from build123d import *

# Parameters (mm, degrees)
F0_R     = 1.25
F1_DEPTH = 2
F2_W     = 20
F2_H     = 3.15
F3_DEPTH = 15
F4_R     = 9.99999
F5_R     = 2.55
F6_DEPTH = 25


# Not quite as in the source:
# - a fillet or chamfer is up to 0.001 mm smaller than in the source, because OpenCascade refuses the exact size


with BuildPart() as f1:
    # F0 (on Top) → F1 (new body)
    with BuildSketch(Plane.XY):
        with BuildLine():
            Line((-33, -15), (33, -15))
            ThreePointArc((33, -15), (34.4142135624, -14.4142135624), (35, -13))
            Line((35, -13), (35, 13))
            ThreePointArc((35, 13), (34.4142135624, 14.4142135624), (33, 15))
            Line((33, 15), (-33, 15))
            ThreePointArc((-33, 15), (-34.4142135624, 14.4142135624), (-35, 13))
            Line((-35, 13), (-35, -13))
            ThreePointArc((-35, -13), (-34.4142135624, -14.4142135624), (-33, -15))
        make_face()
        with Locations((-30.5, -12)):
            Circle(F0_R, mode=Mode.SUBTRACT)
        with Locations((30.5, -12)):
            Circle(F0_R, mode=Mode.SUBTRACT)
        with Locations((-30.5, 12)):
            Circle(F0_R, mode=Mode.SUBTRACT)
        with Locations((30.5, 12)):
            Circle(F0_R, mode=Mode.SUBTRACT)
    extrude(amount=F1_DEPTH)

    # F2 (on face) → F3 (join)
    with BuildSketch(Plane.XY.offset(2)):
        Rectangle(F2_W, F2_H)
        with Locations((0, 6.6)):
            Rectangle(F2_W, F2_H)
        with Locations((0, -6.6)):
            Rectangle(F2_W, F2_H)
    extrude(amount=F3_DEPTH)

    # F4 (radius 10 in the source; OpenCascade refuses exactly that, so slightly less here)
    f4_edges = [f1.edges().sort_by_distance(p)[0] for p in [
        (-10, -6.6, 17),
        (10, -6.6, 17),
        (10, 0, 17),
        (-10, 0, 17),
        (-10, 6.6, 17),
        (10, 6.6, 17),
    ]]
    fillet(f4_edges, radius=F4_R)

    # F5 (on face) → F6 (cut)
    with BuildSketch(Plane.XZ.offset(8.175)):
        with Locations((0, 12)):
            Circle(F5_R)
    extrude(amount=-F6_DEPTH, mode=Mode.SUBTRACT)


solid = f1.part
Work out the finished part from the listing and answer in its coordinate system (mm). A direction names the side the tool comes from. Round coordinates to 2 decimals unless told otherwise and drop trailing zeros. Loops run counter-clockwise (first coordinate to the right, second up) from the corner with the lowest first, then second, coordinate; pieces in that order, holes last. Notation, with made-up numbers: (35.25, 80.5) - (64.25, 80.5) arc R26 ccw to (64.25, 119.5) - close; hole circle Ø5 at (45.5, 2.5). An arc over 180 degrees is marked (long way). Use one line per item in the form item = value. Start each with the question number.
(1) Flat-ended cylindrical pins translate along their axes: P1, Ø4, axis at x = 7, y = 2, coming from the -Z side; P2, Ø4, axis at x = 0, z = 12, coming from the +Y side; P3, Ø8, axis at x = 14, y = 11, coming from the +Z side; P4, Ø3, axis at x = 11, z = 9.5, coming from the +Y side (3 decimals). Find the tip coordinate at first contact, or state that the pin passes through.
(2) Determine the mould class of faces 6 (the face through (0, -5.025, 8)), 7 (the face through (34.4, -14.43, 0.99)), 8 (the face through (7.15, 0.02, 13.99)) for opening direction Y: +Y half, -Y half, draft (parallel to the pull), parting line (faces both ways), or undercut.
(3) Find section B-B on z = 3. Determine the outline of the cut face in (x, y) (3 decimals), and give its area (3 significant figures).
(4) Consider line 1 (Y direction, x = -30.5, z = 1.1); line 2 (Y direction, x = -4, z = 9) (3 decimals); line 3 (Z direction, x = 0, y = 0). Determine where each line is inside the solid, lowest interval first.
(5) Which of the six approach directions +Z, -Z, +X, -X, +Y, -Y give full straight-line access (tool end or side, diameter ignored) to faces 1 (the face through (0, -15, 1)), 2 (the face through (-35, 0, 1)), 3 (the face through (-10, -7, 4)), 4 (the face through (10, 0, 4)), 5 (the face through (0, 1.575, 8))?
(6) Find section C-C on x = -8. Determine the outline of the cut face in (y, z) (3 decimals).
(7) Find section D-D on y = 9. Determine the outline of the cut face in (x, z).
(8) Find section A-A on x = 30.5. Determine the outline of the cut face in (y, z).
Answer list:
q1.P1 = 0
q1.P2 = through
q1.P3 = 2
q1.P4 = 8.175
q2.face_6 = undercut
q2.face_7 = -Y half
q2.face_8 = draft
q3.outline = (-10, -8.175) - (10, -8.175) - (10, -5.025) - (-10, -5.025) - close; (-10, -1.575) - (10, -1.575) - (10, 1.575) - (-10, 1.575) - close; (-10, 5.025) - (10, 5.025) - (10, 8.175) - (-10, 8.175) - close
q3.area = 189 mm^2
q4.line_1 = -15 to -13.25, -10.75 to 10.75, 13.25 to 15
q4.line_2 = -8.175 to -5.025, -1.575 to 1.575, 5.025 to 8.175
q4.line_3 = 0 to 9.45, 14.55 to 17
q5.face_1 = +Z, -Z, +X, -X, -Y
q5.face_2 = +Z, -Z, -X, +Y, -Y
q5.face_3 = +Z, -X, +Y, -Y
q5.face_4 = +Z, +X, +Y, -Y
q5.face_5 = +Z, +X, -X
q6.outline = (-15, 0) - (15, 0) - (15, 2) - (8.175, 2) - (8.175, 13) - (5.025, 13) - (5.025, 2) - (1.575, 2) - (1.575, 13) - (-1.575, 13) - (-1.575, 2) - (-5.025, 2) - (-5.025, 13) - (-8.175, 13) - (-8.175, 2) - (-15, 2) - close
q7.outline = (-35, 0) - (35, 0) - (35, 2) - (-35, 2) - close
q8.outline = (-15, 0) - (-13.25, 0) - (-13.25, 2) - (-15, 2) - close; (-10.75, 0) - (10.75, 0) - (10.75, 2) - (-10.75, 2) - close; (13.25, 0) - (15, 0) - (15, 2) - (13.25, 2) - close
